```python
from build123d import *

# Parameters (mm, degrees)
F0_R     = 8.5
F1_DEPTH = 28
F2_R     = 8.5
F2_W     = 84
F2_H     = 17
F3_DEPTH = 28.001
F4_R     = 13.99999
F5_R     = 5
F6_DEPTH = 54.0266669521


# Not quite as in the source:
# - a fillet or chamfer is up to 0.001 mm smaller than in the source, because OpenCascade refuses the exact size


with BuildPart() as f1:
    # F0 (on Top) → F1 (new body)
    with BuildSketch(Plane.XY):
        with BuildLine():
            Line((41, 14), (-41, 14))
            Line((-41, 14), (-41, 8.5))
            Line((-41, 8.5), (1, 8.5))
            Line((1, 8.5), (1, -8.5))
            Line((1, -8.5), (-41, -8.5))
            Line((-41, -8.5), (-41, -14))
            Line((-41, -14), (41, -14))
            ThreePointArc((41, -14), (55, 0), (41, 14))
        make_face()
        with Locations((41, 0)):
            Circle(F0_R, mode=Mode.SUBTRACT)
    extrude(amount=F1_DEPTH)

    # F2 (on face) → F3 (cut, through all)
    with BuildSketch(Plane.XZ.offset(14)):
        with Locations((-27, 14)):
            Circle(F2_R)
        with Locations((55.0256669521, 14)):
            Rectangle(F2_W, F2_H)
    extrude(amount=-F3_DEPTH, mode=Mode.SUBTRACT)

    # F4 (radius 14 in the source; OpenCascade refuses exactly that, so slightly less here)
    f4_edges = [f1.edges().sort_by_distance(p)[0] for p in [
        (-41, 11.25, 28),
        (-41, 11.25, 0),
        (-41, -11.25, 28),
        (-41, -11.25, 0),
    ]]
    fillet(f4_edges, radius=F4_R)

    # F5 (on face) → F6 (cut, through all)
    with BuildSketch(Plane.YZ.offset(13.0256669521)):
        with Locations((0, 14)):
            Circle(F5_R)
    extrude(amount=-F6_DEPTH, mode=Mode.SUBTRACT)


solid = f1.part
```
Could you check a few things on this model? Use its own coordinates, in mm. A direction names the side the tool comes from. Round coordinates to 2 decimals unless told otherwise and drop trailing zeros. Write each loop counter-clockwise with the first axis right and the second up, starting at its lowest first coordinate (ties: lowest second). Pieces come first, ordered by that corner, then holes. Notation, with made-up numbers: M -6,37.25 L 27,37.25 A34 ccw 27,68.25 Z; hole C 18,-30.75 d10. An arc over 180 degrees is marked long. Write each question's results on one line, items separated by ' | '. Start each with the question number.
1. Imagine slicing it at A-A on y = 0. List the corners of the cut face in (x, z) for me, and give its area (3 significant figures).
2. Imagine slicing it at D-D on y = 7.25. List the corners of the cut face in (x, z) for me.
3. On a 3-axis mill with a long thin cutter (end or side, diameter ignored), from which of +Z, -Z, +X, -X, +Y, -Y can I reach the whole of each face in a straight line? I mean faces 1 (the face through (29, 0, 22.5)), 2 (the face through (34.735, 5.745, 25.212)), 3 (the face through (1, 6, 14)). Say none if no direction works.
4. I'm going to push flat-ended pins straight in: pin 1 Ø13.5 at (x, z) = (-27, 14) entering from -Y; pin 2 Ø13.5 at (y, z) = (0.5, 17.5) entering from -X; pin 3 Ø3 at (y, z) = (4, 10.5) entering from +X; pin 4 Ø6 at (y, z) = (8, 19) entering from -X. Where does each tip first touch, or does it pass through?
5. I need wall thicknesses on L1, parallel to Y at x = -31, z = 24.75; L2, parallel to Z at x = -27, y = -12.5; L3, parallel to Z at x = 9, y = 0. Which ranges of each line are inside material? Lowest first, please. Write a range as from..to.
6. Imagine slicing it at C-C on x = 11.5. List the corners of the cut face in (y, z) for me, and give its area (3 significant figures).
7. Imagine slicing it at B-B on x = -6. List the corners of the cut face in (y, z) for me, and give its area (3 significant figures).
8. Thinking about a two-plate mould opening in X: for faces 4 (the face through (-23.08, 11.21, 6.46)), 5 (the face through (29, 0, 5.5)), 6 (the face through (13.026, 0, 8)), 7 (the face through (-23.08, -11.29, 6.46)), which applies, +X half, -X half, draft (parallel to the pull), parting line (faces both ways), or undercut?
Result sheet:
1) outline: M 1,0 L 32.5,0 L 32.5,5.5 L 13.03,5.5 L 13.03,9 L 1,9 Z; M 1,19 L 13.03,19 L 13.03,22.5 L 32.5,22.5 L 32.5,28 L 1,28 Z; M 49.5,0 L 55,0 L 55,5.5 L 49.5,5.5 Z; M 49.5,22.5 L 55,22.5 L 55,28 L 49.5,28 Z | area: 491 mm^2
2) outline: M 1,0 L 36.56,0 L 36.56,5.5 L 13.03,5.5 L 13.03,22.5 L 36.56,22.5 L 36.56,28 L 1,28 Z; M 45.44,0 L 52.98,0 L 52.98,5.5 L 45.44,5.5 Z; M 45.44,22.5 L 52.98,22.5 L 52.98,28 L 45.44,28 Z
3) face 1: +X, +Y, -Y | face 2: +Z, -Z | face 3: +Z, -Z, -X
4) pin 1: passes through | pin 2: stops at x = 1 | pin 3: stops at x = 13.03 | pin 4: stops at x = -40.85
5) L1: y = -14..-8.5, 8.5..14 | L2: z = 0..5.5, 22.5..28 | L3: z = 0..9, 19..28
6) outline: M -14,0 L 14,0 L 14,28 L -14,28 Z; hole C 0,14 d10 | area: 705 mm^2
7) outline: M -14,0 L -8.5,0 L -8.5,28 L -14,28 Z; M 8.5,0 L 14,0 L 14,28 L 8.5,28 Z | area: 308 mm^2
8) face 4: undercut | face 5: draft | face 6: +X half | face 7: undercut
